from build123d import *

# Parameters (mm, degrees)
SKETCH1_R   = 11.1125
SKETCH1_R_2 = 6.0325
SKETCH1_R_3 = 2.413
SKETCH1_R_4 = 2.6035
PANEL_DEPTH = 1.5875


with BuildPart() as part:
    # Sketch1 → Panel (new body)
    with BuildSketch(Plane.XY):
        Polygon((-233.495394339, -381), (-186.796315472, -304.8), (0, -304.8), (0, -381), align=None)
        with Locations((-171.45, -332.74)):
            Circle(SKETCH1_R, mode=Mode.SUBTRACT)
        with Locations((-196.85, -361.95)):
            Circle(SKETCH1_R_2, mode=Mode.SUBTRACT)
        with Locations((-171.45, -361.95)):
            Circle(SKETCH1_R_2, mode=Mode.SUBTRACT)
        with Locations((-146.05, -361.95)):
            Circle(SKETCH1_R_2, mode=Mode.SUBTRACT)
        with Locations((-6.35, -311.15)):
            Circle(SKETCH1_R_3, mode=Mode.SUBTRACT)
        with Locations((-6.35, -374.65)):
            Circle(SKETCH1_R_3, mode=Mode.SUBTRACT)
        with Locations((-222.156189245, -374.65)):
            Circle(SKETCH1_R_3, mode=Mode.SUBTRACT)
        with Locations((-183.240290189, -311.15)):
            Circle(SKETCH1_R_3, mode=Mode.SUBTRACT)
        with Locations((-19.60215076, -336.167333479)):
            Circle(SKETCH1_R_4, mode=Mode.SUBTRACT)
        with Locations((-56.59784924, -349.632666521)):
            Circle(SKETCH1_R_4, mode=Mode.SUBTRACT)
        with Locations((-83.10215076, -336.167333479)):
            Circle(SKETCH1_R_4, mode=Mode.SUBTRACT)
        with Locations((-120.09784924, -349.632666521)):
            Circle(SKETCH1_R_4, mode=Mode.SUBTRACT)
        with BuildLine():
            Line((-56.904231841, -330.003007558), (-44.214850365, -364.866796631))
            ThreePointArc((-44.214850365, -364.866796631), (-41.786616314, -368.025044915), (-37.983738549, -369.212046828))
            ThreePointArc((-37.983738549, -369.212046828), (-29.099761225, -367.627952805), (-21.276003752, -363.13092868))
            ThreePointArc((-21.276003752, -363.13092868), (-19.125820494, -359.777189752), (-19.295768159, -355.796992442))
            Line((-19.295768159, -355.796992442), (-31.985149635, -320.933203369))
            ThreePointArc((-31.985149635, -320.933203369), (-34.413383686, -317.774955085), (-38.216261451, -316.587953172))
            ThreePointArc((-38.216261451, -316.587953172), (-47.100238775, -318.172047195), (-54.923996248, -322.66907132))
            ThreePointArc((-54.923996248, -322.66907132), (-57.074179506, -326.022810248), (-56.904231841, -330.003007558))
        make_face(mode=Mode.SUBTRACT)
        with BuildLine():
            Line((-120.404231841, -330.003007558), (-107.714850365, -364.866796631))
            ThreePointArc((-107.714850365, -364.866796631), (-105.286616314, -368.025044915), (-101.483738549, -369.212046828))
            ThreePointArc((-101.483738549, -369.212046828), (-92.599761225, -367.627952805), (-84.776003752, -363.13092868))
            ThreePointArc((-84.776003752, -363.13092868), (-82.625820494, -359.777189752), (-82.795768159, -355.796992442))
            Line((-82.795768159, -355.796992442), (-95.485149635, -320.933203369))
            ThreePointArc((-95.485149635, -320.933203369), (-97.913383686, -317.774955085), (-101.716261451, -316.587953172))
            ThreePointArc((-101.716261451, -316.587953172), (-110.600238775, -318.172047195), (-118.423996248, -322.66907132))
            ThreePointArc((-118.423996248, -322.66907132), (-120.574179506, -326.022810248), (-120.404231841, -330.003007558))
        make_face(mode=Mode.SUBTRACT)
    extrude(amount=PANEL_DEPTH)


solid = part.part
The listing builds one solid part. Answer for the finished solid, in the listing's coordinates (mm). Give positions to 0.01 mm unless a question says otherwise; leave off trailing zeros. Write each loop counter-clockwise with the first axis right and the second up, starting at its lowest first coordinate (ties: lowest second). Pieces come first, ordered by that corner, then holes.
1) Section B-B (y = -374.65) is taken. Write down the section's boundary in (x, z).
2) Section A-A (x = -6.35) is taken. Write down the section's boundary in (y, z), and give its area (3 significant figures).
3) Given P1, Ø4.5, axis at x = -6.35, y = -311.15, coming from the -Z side, flat-ended and moving along its own axis, determine where the tip first touches the part or whether it passes through.
4) Section C-C (x = -146.05) is taken. Write down the section's boundary in (y, z).
5) Section D-D (z = 0.3) is taken. Count the separate pieces of the cut face and the enclosed holes in it, and give its area (3 significant figures).
6) Find the intervals of material crossed by L1, parallel to Y at x = -6.35, z = 0.6; L2, parallel to Y at x = -171.45, z = 0.4; L3, parallel to X at y = -338.5, z = 0.85, in increasing order.
7) For a pull along Y with two mould halves and no side action, classify faces 1 (the face through (-115, -351, 1.588)), 2 (the face through (-222.7, -377, 0.8)), 3 (the face through (-172.76, -367.84, 0.78)) as pulls with the +Y half, pulls with the -Y half, needs draft (parallel to the pull), parting line crosses it, or undercut.
Response:
1. outline: (-229.6, 0) - (-224.57, 0) - (-224.57, 1.59) - (-229.6, 1.59) - close; (-219.74, 0) - (-8.76, 0) - (-8.76, 1.59) - (-219.74, 1.59) - close; (-3.94, 0) - (0, 0) - (0, 1.59) - (-3.94, 1.59) - close
2. outline: (-381, 0) - (-377.06, 0) - (-377.06, 1.59) - (-381, 1.59) - close; (-372.24, 0) - (-313.56, 0) - (-313.56, 1.59) - (-372.24, 1.59) - close; (-308.74, 0) - (-304.8, 0) - (-304.8, 1.59) - (-308.74, 1.59) - close
2. area: 106 mm2
3. P1: passes through
4. outline: (-381, 0) - (-367.98, 0) - (-367.98, 1.59) - (-381, 1.59) - close; (-355.92, 0) - (-304.8, 0) - (-304.8, 1.59) - (-355.92, 1.59) - close
5. separate pieces: 1
5. enclosed holes: 14
5. area: 12,500 mm2
6. L1: y = -381 to -377.06, -372.24 to -313.56, -308.74 to -304.8
6. L2: y = -381 to -367.98, -355.92 to -343.85, -321.63 to -304.8
6. L3: x = -207.45 to -180.95, -161.95 to -117.31, -89.09 to -84.26, -81.95 to -53.81, -25.59 to -20.76, -18.45 to 0
7. face 1: needs draft
7. face 2: undercut
7. face 3: undercut
